Autodesk Inventor part; units mm, degrees
ref_plane "YZ Plane" through (0, 0, 0) normal (1, 0, 0) x (0, 1, 0)
ref_plane "XZ Plane" through (0, 0, 0) normal (0, 1, 0) x (-1, 0, 0)
ref_plane "XY Plane" through (0, 0, 0) normal (0, 0, 1) x (1, 0, 0)
sketch "Sketch1" plane through (0, 0, 0) normal (1, 0, 0) x (0, 1, 0)
  line L0 (0, 0) -> (10, 0)
  line L1 (10, 0) -> (10, -25.4)
  line L2 (10, -25.4) -> (0, -25.4)
  line L3 (0, -25.4) -> (0, 0)
  line L4 (5, 0) -> (5, -25.4) construction
  line L5 (10, 0) -> (0, 0)
  line L6 (0, 0) -> (0, -6.35)
  line L7 (0, -6.35) -> (10, -6.35) construction
  line L8 (10, -6.35) -> (10, 0)
  line L9 (10, -25.4) -> (0, -25.4)
  line L10 (0, -25.4) -> (0, -19.05)
  line L11 (0, -19.05) -> (10, -19.05) construction
  line L12 (10, -19.05) -> (10, -25.4)
  circle A0 centre (5, -6.35) radius 1.5875
  circle A1 centre (5, -19.05) radius 1.5875
  line L13 (0, -12.7) -> (-19.05, -12.7)
  line L14 (-9.652, -21.59) -> (-28.448, -21.59)
  line L15 (-28.448, -21.59) -> (-28.448, -3.81)
  line L16 (-28.448, -3.81) -> (-9.652, -3.81)
  line L17 (-9.652, -3.81) -> (-9.652, -21.59)
  line L18 (-9.652, -21.59) -> (-28.448, -3.81) construction
  line L19 (-28.448, -21.59) -> (-9.652, -3.81) construction
  line L20 (-28.448, -3.81) -> (-26.67, -3.81)
  line L21 (-26.67, -3.81) -> (-26.67, -6.096)
  circle A2 centre (-26.67, -6.096) radius 0.635
  circle A3 centre (-26.67, -19.304) radius 0.635
  line L22 (-38.1, 0) -> (0, 0)
  line L23 (0, 0) -> (0, -25.4)
  line L24 (0, -25.4) -> (-38.1, -25.4)
  line L25 (-38.1, -25.4) -> (-38.1, 0)
  line L26 (-38.1, 0) -> (0, -25.4) construction
  line L27 (0, 0) -> (-38.1, -25.4) construction
  dimension "d0" = 10
  dimension "d1" = 25.4
  dimension "d2" = 6.35
  dimension "d3" = 6.35
  dimension "d4" = 3.175
  dimension "d5" = 3.175
  dimension "d6" = 19.05
  dimension "d7" = 18.796
  dimension "d8" = 17.78
  dimension "d9" = 1.778
  dimension "d10" = 2.286
  dimension "d11" = 1.27
extrude "Extrusion1" add sketch "Sketch1" along normal blind 7.5 contours L0 L1 L2 L3 | L17 L14 L15 L16 | L3 L24 L25 L22
sketch "Sketch2" plane through (7.5, 0, 0) normal (1, 0, 0) x (0, 0, -1)
  circle A0 centre (19.304, -26.67) radius 0.635
  circle A1 centre (6.096, -26.67) radius 0.635
  circle A2 centre (19.05, 5) radius 1.5875
  circle A3 centre (6.35, 5) radius 1.5875
  line L0 (25.4, -38.1) -> (25.4, 10)
  line L1 (25.4, 10) -> (0, 10)
  line L2 (0, 10) -> (0, -38.1)
  line L3 (0, -38.1) -> (25.4, -38.1)
  line L4 (25.4, 10) -> (0, 10)
  line L5 (3.175, 0) -> (22.225, 0)
  line L6 (22.225, 0) -> (22.225, 10)
  line L7 (22.225, 10) -> (3.175, 10)
  line L8 (3.175, 10) -> (3.175, 0)
  line L9 (3.175, 0) -> (22.225, 10) construction
  line L10 (22.225, 0) -> (3.175, 10) construction
  line L11 (25.4, -38.1) -> (25.4, 10)
  line L12 (0, 0) -> (25.4, 0)
  line L13 (25.4, 0) -> (25.4, 10)
  line L14 (25.4, 10) -> (0, 10)
  line L15 (0, 10) -> (0, 0)
  line L16 (0, 0) -> (25.4, 10) construction
  line L17 (25.4, 0) -> (0, 10) construction
  point P0 (12.7, 5)
  dimension "d14" = 19.05
extrude "Extrusion2" cut sketch "Sketch2" against normal blind 7.5 contours L12 L6 L1 L0 | L2 L1 L8 L12
properties part number "magMount" material "Polyethylene, High Density"
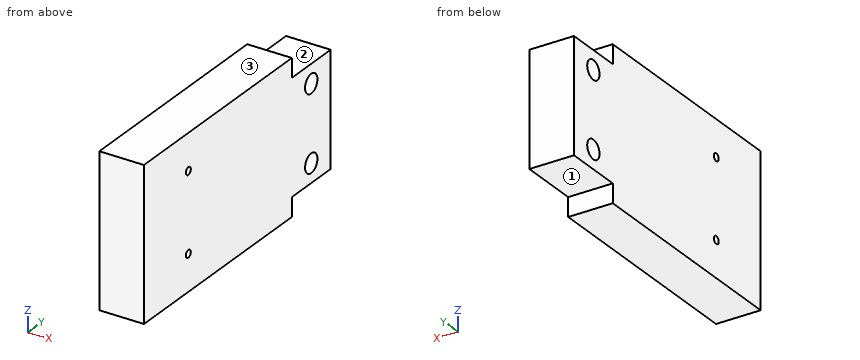
Work out the finished part from the listing and answer in its coordinate system (mm). Face numbers are marked on the shaded views. A direction names the side the tool comes from. Round coordinates to 2 decimals unless told otherwise and drop trailing zeros. Write each loop counter-clockwise with the first axis right and the second up, starting at its lowest first coordinate (ties: lowest second). Pieces come first, ordered by that corner, then holes.
1) A cutting plane is placed at C-C on y = 5. Determine the outline of the cut face in (x, z) (1 decimal), and give its area (4 significant figures).
2) Consider probe 1 along Z at (x, y) = (3.25, 5) (1 decimal); probe 2 along Z at (x, y) = (2.75, -26.67); probe 3 along Y at (x, z) = (6, -6.5). Determine where each line is inside the solid, lowest interval first.
3) Which of the six approach directions +Z, -Z, +X, -X, +Y, -Y give full straight-line access (tool end or side, diameter ignored) to the marked faces 1, 2 and 3?
4) A cutting plane is placed at B-B on x = 2.25. Give the number of separate pieces and of enclosed holes in the cut face, and give its area (3 significant figures).
5) A cutting plane is placed at D-D on z = -1.75. Determine the outline of the cut face in (x, y), and give its area (3 significant figures).
6) A cutting plane is placed at A-A on y = -26.67. Determine the outline of the cut face in (x, z), and give its area (3 significant figures).
7) Flat-ended cylindrical pins translate along their axes: P1, Ø2.5, axis at x = 5.5, z = -1.5, coming from the +Y side; P2, Ø2.5, axis at y = 5, z = -6.35, coming from the -X side. Find the tip coordinate at first contact, or state that the pin passes through.
Entries:
1. outline: (0, -22.2) - (7.5, -22.2) - (7.5, -20.6) - (0, -20.6) - close; (0, -17.5) - (7.5, -17.5) - (7.5, -7.9) - (0, -7.9) - close; (0, -4.8) - (7.5, -4.8) - (7.5, -3.2) - (0, -3.2) - close
1. area: 95.25 mm2
2. probe 1: z = -22.2 to -20.6, -17.5 to -7.9, -4.8 to -3.2
2. probe 2: z = -25.4 to -19.94, -18.67 to -6.73, -5.46 to 0
2. probe 3: y = -38.1 to -27.16, -26.18 to 3.42, 6.58 to 10
3. face 1: -Z, +X, -X, +Y
3. face 2: +Z, +X, -X, +Y
3. face 3: +Z, +X, -X, +Y, -Y
4. separate pieces: 1
4. enclosed holes: 4
4. area: 1,140 mm2
5. outline: (0, -38.1) - (7.5, -38.1) - (7.5, 0) - (0, 0) - close
5. area: 286 mm2
6. outline: (0, -25.4) - (7.5, -25.4) - (7.5, -19.94) - (0, -19.94) - close; (0, -18.67) - (7.5, -18.67) - (7.5, -6.73) - (0, -6.73) - close; (0, -5.46) - (7.5, -5.46) - (7.5, 0) - (0, 0) - close
6. area: 171 mm2
7. P1: stops at y = 0
7. P2: passes through
